```python
from build123d import *

# Parameters (mm, degrees)
SKETCH1_W           = 3.175
SKETCH1_H           = 50.8
BOSS_EXTRUDE1_DEPTH = 25.4
SKETCH2_R           = 6.35
BOSS_EXTRUDE2_DEPTH = 6.35


with BuildPart() as part:
    # Sketch1 → Boss-Extrude1 (new body)
    with BuildSketch(Plane.XY):
        with Locations((-1.5875, 25.4)):
            Rectangle(SKETCH1_W, SKETCH1_H)
    extrude(amount=BOSS_EXTRUDE1_DEPTH)

    # Sketch2 → Boss-Extrude2 (add)
    with BuildSketch(Plane.ZY.offset(3.175)):
        with Locations(Location((12.7, 40.386207141, 0), (0, 0, 180))):
            Circle(SKETCH2_R)
    extrude(amount=BOSS_EXTRUDE2_DEPTH)

    # Sketch5 → Revolve2 (revolve)
    with BuildSketch(Plane.XY.offset(12.7)):
        Polygon((0, 43.146240345), (11.795403193, 36.336161137), (10.207903193, 33.586530479), (0, 39.480066136), align=None)
    revolve(axis=Axis((10.207903193, 33.586530479, 12.7), (-0.8660254037844417, 0.4999999999999948, 0)))


solid = part.part
```
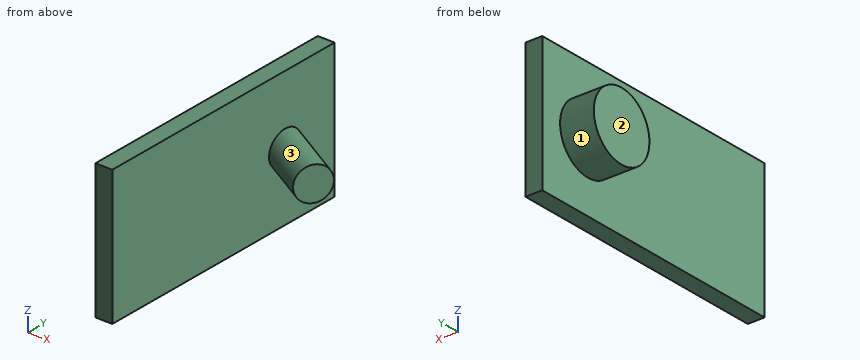
Can you work these out from the model? Positions are in its coordinate system, mm. Face numbers are marked on the shaded views. Round coordinates to 2 decimals unless told otherwise and drop trailing zeros. Loops run counter-clockwise (first coordinate to the right, second up) from the corner with the lowest first, then second, coordinate; pieces in that order, holes last.
Item 1: Will these pins go through, and if not, where does the flat tip stop? pin 1 Ø4 at (y, z) = (13.5, 10) entering from -X (3 decimals); pin 2 Ø1 at (y, z) = (13.5, 6.5) entering from +X.
Item 2: Please list where these lines run through material, in increasing order: L1, parallel to X at y = 29.5, z = 12.25 (3 decimals); L2, parallel to Z at x = 3.25, y = 34.5; L3, parallel to Z at x = -4, y = 46.
Item 3: Suppose I cut it at D-D, the plane z = 20.5. Write out the boundary of the cut face in (x, y) (3 decimals).
Item 4: Suppose I cut it at A-A, the plane z = 7. Write out the boundary of the cut face in (x, y) (3 decimals).
Item 5: Suppose I cut it at B-B, the plane y = 28. Write out the boundary of the cut face in (x, z) (3 decimals), then the cut area to 3 significant figures.
Item 6: Suppose I cut it at C-C, the plane z = 11.5. Write out the boundary of the cut face in (x, y) (3 decimals).
Item 7: If we mould it in two halves opening along X, with no side actions, what happens to the marked faces 1, 2 and 3? For each: +X half, -X half, draft (parallel to the pull), parting line (faces both ways), or undercut.
Reported:
1. pin 1: stops at x = -3.175
1. pin 2: stops at x = 0
2. L1: x = -3.175 to 0
2. L2: z = 11.01 to 14.39
2. L3: z = 9.73 to 15.67
3. outline: (-3.175, 0) - (0, 0) - (0, 50.8) - (-3.175, 50.8) - close
4. outline: (-9.525, 37.588) - (-3.175, 37.588) - (-3.175, 0) - (0, 0) - (0, 50.8) - (-3.175, 50.8) - (-3.175, 43.185) - (-9.525, 43.185) - close
5. outline: (-3.175, 0) - (0, 0) - (0, 25.4) - (-3.175, 25.4) - close
5. area: 80.6 mm2
6. outline: (-9.525, 34.151) - (-3.175, 34.151) - (-3.175, 0) - (0, 0) - (0, 36.086) - (8.738, 31.041) - (11.678, 36.132) - (0, 42.874) - (0, 50.8) - (-3.175, 50.8) - (-3.175, 46.622) - (-9.525, 46.622) - close
7. face 1: draft
7. face 2: -X half
7. face 3: undercut
